CAD build for the part. Positions are in the model's coordinates, mm. A direction names the side the tool comes from. Round coordinates to 2 decimals unless told otherwise and drop trailing zeros. Order: outer loops, then holes, each group sorted by start corner. A loop starts at its lowest first (then second) coordinate and runs counter-clockwise, first axis right, second up. Notation, with made-up numbers: (25, 69) -> (49, 69) arc R13 ccw to (49, 86) -> close; hole circle Ø7 at (-28.5, -37). An arc over 180 degrees is marked (long way). Answer as CSV lines item,"result". Start each with the question number.
from build123d import *

# Parameters (mm, degrees)
SKETCH1_W           = 98.425
SKETCH1_H           = 98.425
BOSS_EXTRUDE1_DEPTH = 4.7625
CUT_EXTRUDE1_REACH  = 119.54
SKETCH4_R           = 1.27
SKETCH4_R_2         = 1.905
SKETCH4_W           = 75.692
SKETCH4_H           = 31.496
CUT_EXTRUDE2_REACH  = 119.54
SKETCH5_W           = 4.5085
SKETCH5_H           = 7.3025
FILLET1_R           = 2.54
FILLET3_R           = 2.54
FILLET4_R           = 2.54


with BuildPart() as part:
    # Sketch1 → Boss-Extrude1 (new body)
    with BuildSketch(Plane.XY):
        with Locations((-38.559564005, 28.819230769)):
            Rectangle(SKETCH1_W, SKETCH1_H)
    extrude(amount=BOSS_EXTRUDE1_DEPTH)

    # Sketch4 → Cut-Extrude1 (cut, up to next)
    with BuildSketch(Plane(origin=(0, 0, 0), x_dir=(-1, 0, 0), z_dir=(0, 0, -1)), mode=Mode.PRIVATE) as cut_extrude1_sk1:
        with Locations(Location((72.341564005, 55.870230769, 0), (0, 0, 180))):
            Circle(SKETCH4_R)
    cut_extrude1_tool1 = extrude(cut_extrude1_sk1.sketch, amount=-CUT_EXTRUDE1_REACH, mode=Mode.PRIVATE) & part.part
    # Sketch4 → Cut-Extrude1 (cut, up to next)
    with BuildSketch(Plane(origin=(0, 0, 0), x_dir=(-1, 0, 0), z_dir=(0, 0, -1)), mode=Mode.PRIVATE) as cut_extrude1_sk2:
        with Locations((72.341564005, 1.768230769)):
            Circle(SKETCH4_R)
    cut_extrude1_tool2 = extrude(cut_extrude1_sk2.sketch, amount=-CUT_EXTRUDE1_REACH, mode=Mode.PRIVATE) & part.part
    # Sketch4 → Cut-Extrude1 (cut, up to next)
    with BuildSketch(Plane(origin=(0, 0, 0), x_dir=(-1, 0, 0), z_dir=(0, 0, -1)), mode=Mode.PRIVATE) as cut_extrude1_sk3:
        with Locations((4.777564005, 55.870230769)):
            Circle(SKETCH4_R)
    cut_extrude1_tool3 = extrude(cut_extrude1_sk3.sketch, amount=-CUT_EXTRUDE1_REACH, mode=Mode.PRIVATE) & part.part
    # Sketch4 → Cut-Extrude1 (cut, up to next)
    with BuildSketch(Plane(origin=(0, 0, 0), x_dir=(-1, 0, 0), z_dir=(0, 0, -1)), mode=Mode.PRIVATE) as cut_extrude1_sk4:
        with Locations(Location((4.777564005, 1.768230769, 0), (0, 0, 180))):
            Circle(SKETCH4_R)
    cut_extrude1_tool4 = extrude(cut_extrude1_sk4.sketch, amount=-CUT_EXTRUDE1_REACH, mode=Mode.PRIVATE) & part.part
    # Sketch4 → Cut-Extrude1 (cut, up to next)
    with BuildSketch(Plane(origin=(0, 0, 0), x_dir=(-1, 0, 0), z_dir=(0, 0, -1)), mode=Mode.PRIVATE) as cut_extrude1_sk5:
        with Locations((-6.080935995, 73.459730769)):
            Circle(SKETCH4_R_2)
    cut_extrude1_tool5 = extrude(cut_extrude1_sk5.sketch, amount=-CUT_EXTRUDE1_REACH, mode=Mode.PRIVATE) & part.part
    # Sketch4 → Cut-Extrude1 (cut, up to next)
    with BuildSketch(Plane(origin=(0, 0, 0), x_dir=(-1, 0, 0), z_dir=(0, 0, -1)), mode=Mode.PRIVATE) as cut_extrude1_sk6:
        with Locations(Location((83.200064005, 73.459730769, 0), (0, 0, 180))):
            Circle(SKETCH4_R_2)
    cut_extrude1_tool6 = extrude(cut_extrude1_sk6.sketch, amount=-CUT_EXTRUDE1_REACH, mode=Mode.PRIVATE) & part.part
    # Sketch4 → Cut-Extrude1 (cut, up to next)
    with BuildSketch(Plane(origin=(0, 0, 0), x_dir=(-1, 0, 0), z_dir=(0, 0, -1)), mode=Mode.PRIVATE) as cut_extrude1_sk7:
        with Locations((-2.334435995, -17.218269231)):
            Circle(SKETCH4_R_2)
    cut_extrude1_tool7 = extrude(cut_extrude1_sk7.sketch, amount=-CUT_EXTRUDE1_REACH, mode=Mode.PRIVATE) & part.part
    # Sketch4 → Cut-Extrude1 (cut, up to next)
    with BuildSketch(Plane(origin=(0, 0, 0), x_dir=(-1, 0, 0), z_dir=(0, 0, -1)), mode=Mode.PRIVATE) as cut_extrude1_sk8:
        with Locations((79.453564005, -17.218269231)):
            Circle(SKETCH4_R_2)
    cut_extrude1_tool8 = extrude(cut_extrude1_sk8.sketch, amount=-CUT_EXTRUDE1_REACH, mode=Mode.PRIVATE) & part.part
    # Sketch4 → Cut-Extrude1 (cut, up to next)
    with BuildSketch(Plane(origin=(0, 0, 0), x_dir=(-1, 0, 0), z_dir=(0, 0, -1)), mode=Mode.PRIVATE) as cut_extrude1_sk9:
        with Locations((38.559564005, 28.819230769)):
            Rectangle(SKETCH4_W, SKETCH4_H)
    cut_extrude1_tool9 = extrude(cut_extrude1_sk9.sketch, amount=-CUT_EXTRUDE1_REACH, mode=Mode.PRIVATE) & part.part
    add(cut_extrude1_tool1.solids().sort_by_distance((-72.341564, 55.870231, 0))[0], mode=Mode.SUBTRACT)
    add(cut_extrude1_tool2.solids().sort_by_distance((-72.341564, 1.768231, 0))[0], mode=Mode.SUBTRACT)
    add(cut_extrude1_tool3.solids().sort_by_distance((-4.777564, 55.870231, 0))[0], mode=Mode.SUBTRACT)
    add(cut_extrude1_tool4.solids().sort_by_distance((-4.777564, 1.768231, 0))[0], mode=Mode.SUBTRACT)
    add(cut_extrude1_tool5.solids().sort_by_distance((6.080936, 73.459731, 0))[0], mode=Mode.SUBTRACT)
    add(cut_extrude1_tool6.solids().sort_by_distance((-83.200064, 73.459731, 0))[0], mode=Mode.SUBTRACT)
    add(cut_extrude1_tool7.solids().sort_by_distance((2.334436, -17.218269, 0))[0], mode=Mode.SUBTRACT)
    add(cut_extrude1_tool8.solids().sort_by_distance((-79.453564, -17.218269, 0))[0], mode=Mode.SUBTRACT)
    add(cut_extrude1_tool9.solids().sort_by_distance((-38.559564, 28.819231, 0))[0], mode=Mode.SUBTRACT)

    # Sketch5 → Cut-Extrude2 (cut, up to next)
    with BuildSketch(Plane(origin=(0, 0, 0), x_dir=(-1, 0, 0), z_dir=(0, 0, -1)), mode=Mode.PRIVATE) as cut_extrude2_sk1:
        with Locations((-8.398685995, -16.742019231)):
            Rectangle(SKETCH5_W, SKETCH5_H)
    cut_extrude2_tool1 = extrude(cut_extrude2_sk1.sketch, amount=-CUT_EXTRUDE2_REACH, mode=Mode.PRIVATE) & part.part
    # Sketch5 → Cut-Extrude2 (cut, up to next)
    with BuildSketch(Plane(origin=(0, 0, 0), x_dir=(-1, 0, 0), z_dir=(0, 0, -1)), mode=Mode.PRIVATE) as cut_extrude2_sk2:
        with Locations((85.517814005, -16.742019231)):
            Rectangle(SKETCH5_W, SKETCH5_H)
    cut_extrude2_tool2 = extrude(cut_extrude2_sk2.sketch, amount=-CUT_EXTRUDE2_REACH, mode=Mode.PRIVATE) & part.part
    add(cut_extrude2_tool1.solids().sort_by_distance((8.398686, -16.742019, 0))[0], mode=Mode.SUBTRACT)
    add(cut_extrude2_tool2.solids().sort_by_distance((-85.517814, -16.742019, 0))[0], mode=Mode.SUBTRACT)

    # Fillet1
    fillet1_edges = [part.edges().sort_by_distance(p)[0] for p in [
        (-87.772064005, 78.031730769, 2.38125),
        (10.652935995, 78.031730769, 2.38125),
    ]]
    fillet(fillet1_edges, radius=FILLET1_R)

    # Fillet3
    fillet3_edges = [part.edges().sort_by_distance(p)[0] for p in [
        (-0.713564005, 13.071230769, 2.38125),
        (-0.713564005, 44.567230769, 2.38125),
        (-76.405564005, 44.567230769, 2.38125),
        (-76.405564005, 13.071230769, 2.38125),
    ]]
    fillet(fillet3_edges, radius=FILLET3_R)

    # Fillet4
    fillet4_edges = [part.edges().sort_by_distance(p)[0] for p in [
        (6.144435995, -20.393269231, 2.38125),
        (10.652935995, -13.090769231, 2.38125),
        (-83.263564005, -20.393269231, 2.38125),
        (-87.772064005, -13.090769231, 2.38125),
    ]]
    fillet(fillet4_edges, radius=FILLET4_R)


solid = part.part
Item 1: Band-saw the part on C-C, the plane z = 2.6. Count the separate pieces of the cut face and the enclosed holes in it, and give its area (3 significant figures).
Item 2: Band-saw the part on A-A, the plane x = -38.5. Give the cut face in (y, z), and give its area (3 significant figures).
Item 3: Probe line 1 (X direction, y = 56, z = 4.4); line 2 (Y direction, x = -40, z = 1.5); line 3 (X direction, y = 33, z = 4.35). List the from-to ranges inside material, lowest first.
Item 4: Mould opens along X. For faces 4 (the cylindrical face through (5.38, -19.67, 2.41)), 5 (the cylindrical face through (-82.54, -19.63, 2.41)), 6 (the cylindrical face through (2.58, -15.33, 2.35)) say: released by +X, released by -X, zero draft, split by the parting line, or undercut.
Item 5: Pin check, flat tips, straight feed: pin 1 (1.5 mm diameter, centred on x = -72.34, y = 55.87, fed in from +Z); pin 2 (1.6 mm diameter, centred on x = -84.5, z = 3, fed in from -Y). Stop position of each tip, or through.
Item 6: Tool access for faces 1 (the flat face through (-38, 44.567, 2)), 2 (the cylindrical face through (9.889, 77.307, 2.415)), 3 (the flat face through (6.144, -16, 2)): list every direction of +Z, -Z, +X, -X, +Y, -Y with a clear straight run to the whole face (end or side of a thin tool).
Item 7: Band-saw the part on B-B, the plane y = 29. Give the cut face in (x, z).
Values:
1,separate pieces,"1"
1,enclosed holes,"9"
1,area,"7,170 mm²"
2,outline,"(-20.39, 0) -> (13.07, 0) -> (13.07, 4.76) -> (-20.39, 4.76) -> close; (44.57, 0) -> (78.03, 0) -> (78.03, 4.76) -> (44.57, 4.76) -> close"
2,area,"319 mm²"
3,line 1,"-87.77 to -73.6, -71.08 to -6.04, -3.51 to 10.65"
3,line 2,"-20.39 to 13.07, 44.57 to 78.03"
3,line 3,"-87.77 to -76.41, -0.71 to 10.65"
4,face 4,"released by +X"
4,face 5,"released by -X"
4,face 6,"undercut"
5,pin 1,"through"
5,pin 2,"y = -13.09"
6,face 1,"+Z, -Z"
6,face 2,"+Z, -Z, +X, +Y"
6,face 3,"+Z, -Z, +X, -Y"
7,outline,"(-87.77, 0) -> (-76.41, 0) -> (-76.41, 4.76) -> (-87.77, 4.76) -> close; (-0.71, 0) -> (10.65, 0) -> (10.65, 4.76) -> (-0.71, 4.76) -> close"
